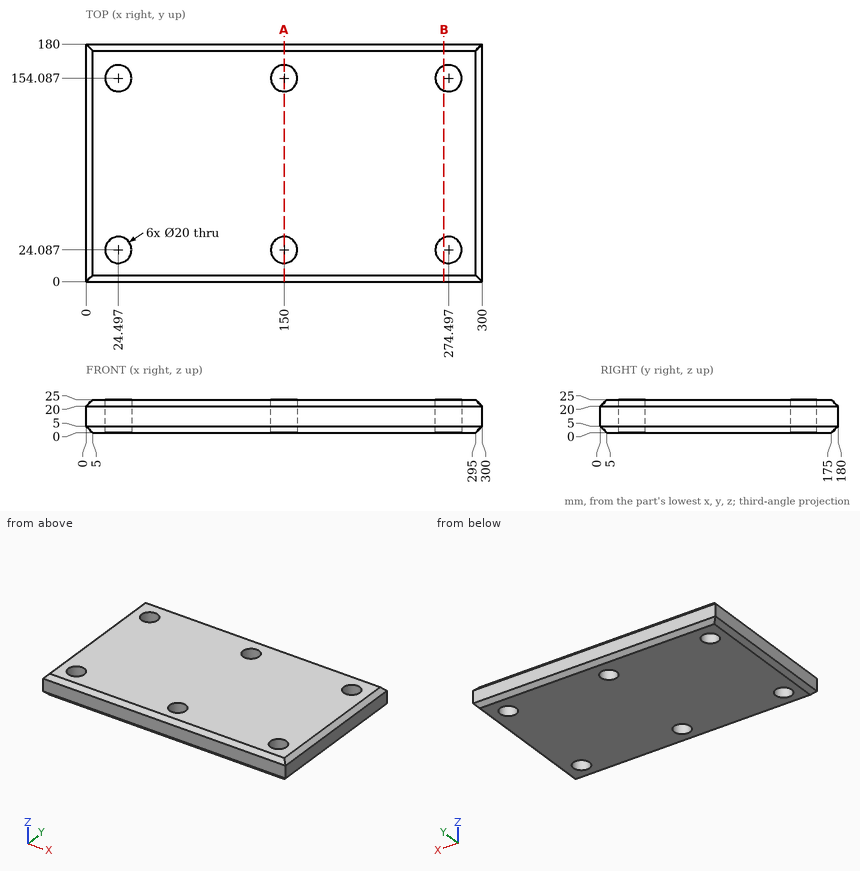
Input: dimensioned drawing with shaded views. Units: mm. Origin: part minimum x, y, z. Coordinates: 2 decimals unless noted, no trailing zeros. Loops run counter-clockwise (first coordinate to the right, second up) from the corner with the lowest first, then second, coordinate; pieces in that order, holes last. Notation, with made-up numbers: (57.25, -1.5) -> (84.25, -1.5) arc R12 cw to (84.25, 16.5) -> close; hole circle Ø8 at (74, -6.5). An arc over 180 degrees is marked (long way). Use a Markdown table: item, result. Add a question column.
(1) Pin query (flat end, axial travel): pin 1 Ø2 at (x, y) = (142.5, 151.5) entering from +Z (1 decimal). Return the tip coordinate at first contact, or that it passes through.
(2) Section query A-A, the plane x = 150. Return loops of the section in (y, z).
(3) Section query B-B, the plane x = 271. Return loops of the section in (y, z), plus the area to 3 significant figures.
(4) Line query: line 1 along X through (y, z) = (32, 13.75) (1 decimal); line 2 along X through (y, z) = (160, 10) (1 decimal); line 3 along Y through (x, z) = (22, 12) (1 decimal). Output: solid intervals per line, ascending.
Answer:
| question | item | result |
|---|---|---|
| 1 | pin 1 | passes through |
| 2 | outline | (0, 5) -> (5, 0) -> (14.09, 0) -> (14.09, 25) -> (5, 25) -> (0, 20) -> close; (34.09, 0) -> (144.09, 0) -> (144.09, 25) -> (34.09, 25) -> close; (164.09, 0) -> (175, 0) -> (180, 5) -> (180, 20) -> (175, 25) -> (164.09, 25) -> close |
| 3 | outline | (0, 5) -> (5, 0) -> (14.72, 0) -> (14.72, 25) -> (5, 25) -> (0, 20) -> close; (33.46, 0) -> (144.72, 0) -> (144.72, 25) -> (33.46, 25) -> close; (163.46, 0) -> (175, 0) -> (180, 5) -> (180, 20) -> (175, 25) -> (163.46, 25) -> close |
| 3 | area | 3,510 mm^2 |
| 4 | line 1 | x = 0 to 18.4, 30.6 to 143.9, 156.1 to 268.4, 280.6 to 300 |
| 4 | line 2 | x = 0 to 16.4, 32.6 to 141.9, 158.1 to 266.4, 282.6 to 300 |
| 4 | line 3 | y = 0 to 14.4, 33.8 to 144.4, 163.8 to 180 |
